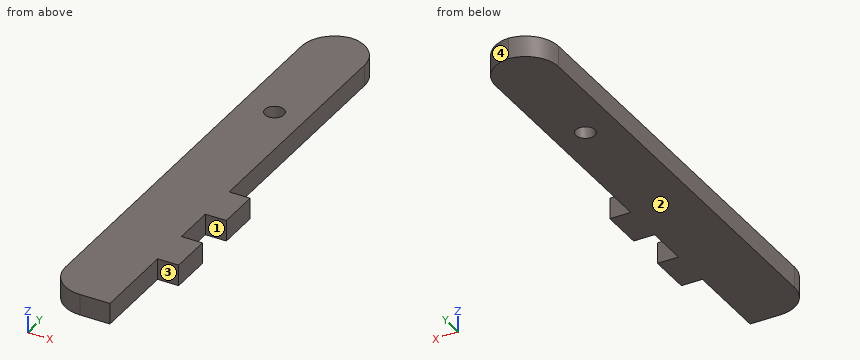
```python
from build123d import *

# Parameters (mm, degrees)
BOSS_EXTRUDE1_DEPTH = 6.35
FILLET1_R           = 10
SKETCH2_R           = 2.8702
CUT_EXTRUDE3_DEPTH  = 120.57148989


with BuildPart() as part:
    # Sketch1 → Boss-Extrude1 (new body)
    with BuildSketch(Plane.XY):
        Polygon((-44.45, 19.05), (-44.45, 101.128885963), (-63.5, 101.128885963), (-63.5, -44.45), (-44.45, -44.45), (-44.45, -19.05), (-38.1, -19.05), (-38.1, -6.35), (-44.45, -6.35), (-44.45, 6.35), (-38.1, 6.35), (-38.1, 19.05), align=None)
    extrude(amount=BOSS_EXTRUDE1_DEPTH)

    # Fillet1
    # the kernel refuses this fillet: 10 mm, written as the material it takes off along each edge
    with BuildSketch(Plane(origin=(-63.5, -44.45, -25), x_dir=(0, 1, 0), z_dir=(0, 0, 1)), Plane(origin=(-44.45, 101.128885963, -25), x_dir=(0, -1, 0), z_dir=(0, 0, 1)), Plane(origin=(-63.5, 101.128885963, -25), x_dir=(1, 0, 0), z_dir=(0, 0, 1))) as fillet1_piece_1:
        with BuildLine():
            CenterArc((FILLET1_R, -FILLET1_R), FILLET1_R, 90, 90)
            Line((0, -FILLET1_R), (0, 0))
            Line((0, 0), (FILLET1_R, 0))
        make_face()
    extrude(amount=56.35, mode=Mode.SUBTRACT)

    # Sketch2 → Cut-Extrude3 (cut, through all)
    with BuildSketch(Plane(origin=(0, 0, 0), x_dir=(-1, 0, 0), z_dir=(0, 0, -1))):
        with Locations((53.575, 59.289941788)):
            Circle(SKETCH2_R)
    extrude(amount=-CUT_EXTRUDE3_DEPTH, mode=Mode.SUBTRACT)


solid = part.part
```
Read the model definition and answer for the solid it produces. Units are mm, in the model's axes. Face numbers are marked on the shaded views. Coordinates: 2 decimals unless noted, no trailing zeros. Loops run counter-clockwise (first coordinate to the right, second up) from the corner with the lowest first, then second, coordinate; pieces in that order, holes last. Notation, with made-up numbers: (38, 73.5) - (78, 73.5) arc R13 ccw to (78, 92.5) - close; hole circle Ø3 at (-34.5, 22.25). An arc over 180 degrees is marked (long way). Answer in a Markdown table with one row per item.
1. Straight lines are drawn through the part: line 1 (Y direction, x = -43.25, z = 3); line 2 (X direction, y = 87, z = 0.75); line 3 (Y direction, x = -51.75, z = 1.5). For each, find the intervals that lie inside material, in ascending order.
Conclusion:
| item | result |
|---|---|
| line 1 | y = -19.05 to -6.35, 6.35 to 19.05 |
| line 2 | x = -63.5 to -44.45 |
| line 3 | y = -44.45 to 57.07, 61.51 to 100.76 |
2. Find section B-B, the plane z = 2.25. Write down the section's boundary in (x, y) (3 decimals), then the cut area to 3 significant figures.
Conclusion:
| item | result |
|---|---|
| outline | (-63.5, -34.45) arc R10 ccw to (-53.5, -44.45) - (-44.45, -44.45) - (-44.45, -19.05) - (-38.1, -19.05) - (-38.1, -6.35) - (-44.45, -6.35) - (-44.45, 6.35) - (-38.1, 6.35) - (-38.1, 19.05) - (-44.45, 19.05) - (-44.45, 91.129) arc R10 ccw to (-53.975, 101.118) arc R10 ccw to (-63.5, 91.129) - close; hole circle Ø5.74 at (-53.575, 59.29) |
| area | 2,840 mm² |
3. Determine the mould class of the marked faces 1, 2, 3 and 4 for opening direction Y: +Y half, -Y half, draft (parallel to the pull), parting line (faces both ways), or undercut.
Conclusion:
| item | result |
|---|---|
| face 1 | undercut |
| face 2 | draft |
| face 3 | -Y half |
| face 4 | +Y half |
4. Find section D-D, the plane x = -46.25. Write down the section's boundary in (y, z), then the cut area to 3 significant figures.
Conclusion:
| item | result |
|---|---|
| outline | (-44.45, 0) - (96.85, 0) - (96.85, 6.35) - (-44.45, 6.35) - close |
| area | 897 mm² |
5. Given pin 1 (3 mm diameter, centred on x = -42.5, z = 2.5, fed in from -Y); pin 2 (1.9 mm diameter, centred on y = -26.5, z = 2.5, fed in from +X); pin 3 (1 mm diameter, centred on x = -49, z = 1, fed in from +Y); pin 4 (4.5 mm diameter, centred on x = -53.58, y = 59.29, fed in from +Z), each flat-ended and moving along its own axis, determine where each tip first touches the part or whether it passes through.
Conclusion:
| item | result |
|---|---|
| pin 1 | stops at y = -19.05 |
| pin 2 | stops at x = -44.45 |
| pin 3 | stops at y = 99.82 |
| pin 4 | passes through |
6. Find section C-C, the plane y = 0. Write down the section's boundary in (x, z), then the cut area to 3 significant figures.
Conclusion:
| item | result |
|---|---|
| outline | (-63.5, 0) - (-44.45, 0) - (-44.45, 6.35) - (-63.5, 6.35) - close |
| area | 121 mm² |
7. Find section A-A, the plane x = -39.75. Write down the section's boundary in (y, z).
Conclusion:
| item | result |
|---|---|
| outline | (-19.05, 0) - (-6.35, 0) - (-6.35, 6.35) - (-19.05, 6.35) - close; (6.35, 0) - (19.05, 0) - (19.05, 6.35) - (6.35, 6.35) - close |
